from build123d import *

# Parameters (mm, degrees)
ESBO_O1_W                = 300
ESBO_O1_H                = 25
RESSALTO_EXTRUS_O1_DEPTH = 2
ESBO_O2_R                = 2.5
CORTE_EXTRUS_O1_DEPTH    = 3
ESBO_O3_W                = 300
ESBO_O3_H                = 2
RESSALTO_EXTRUS_O2_DEPTH = 25
FILETE1_R                = 3


with BuildPart() as part:
    # Esboço1 → Ressalto-extrusão1 (new body)
    with BuildSketch(Plane(origin=(0, 0, 0), x_dir=(1, 0, 0), z_dir=(0, 1, 0))):
        Rectangle(ESBO_O1_W, ESBO_O1_H)
    extrude(amount=RESSALTO_EXTRUS_O1_DEPTH)

    # Esboço2 → Corte-extrusão1 (cut, through all)
    with BuildSketch(Plane(origin=(0, 2, 0), x_dir=(1, 0, 0), z_dir=(0, 1, 0))):
        with Locations((-130, -2.5)):
            Circle(ESBO_O2_R)
        with Locations((-65, -2.5)):
            Circle(ESBO_O2_R)
        with Locations((0, -2.5)):
            Circle(ESBO_O2_R)
        with Locations((65, -2.5)):
            Circle(ESBO_O2_R)
        with Locations((130, -2.5)):
            Circle(ESBO_O2_R)
    extrude(amount=-CORTE_EXTRUS_O1_DEPTH, mode=Mode.SUBTRACT)

    # Esboço3 → Ressalto-extrusão2 (add)
    with BuildSketch(Plane.XZ):
        with Locations((0, -11.5)):
            Rectangle(ESBO_O3_W, ESBO_O3_H)
    extrude(amount=RESSALTO_EXTRUS_O2_DEPTH)

    # Filete1
    filete1_edges = [part.edges().sort_by_distance(p)[0] for p in [
        (0, 2, -12.5),
    ]]
    fillet(filete1_edges, radius=FILETE1_R)


solid = part.part
Here's how the part is built. I have some questions about the finished solid (model axes, mm). A direction names the side the tool comes from. Coordinates: 2 decimals unless noted, no trailing zeros. Write each loop counter-clockwise with the first axis right and the second up, starting at its lowest first coordinate (ties: lowest second). Pieces come first, ordered by that corner, then holes.
Item 1: If we mould it in two halves opening along X, with no side actions, what happens to faces 1 (the cylindrical face through (-127.615, 1.014, 1.749)), 2 (the flat face through (150, -5, -11)), 3 (the flat face through (-2, 2, -1)), 4 (the flat face through (-150, -5, -11))? For each: +X half, -X half, draft (parallel to the pull), parting line (faces both ways), or undercut.
Item 2: If I drill on line 1 (X direction, y = 0.9, z = 2.5); line 2 (Z direction, x = -92.5, y = -23); line 3 (Y direction, x = 82, z = 0.5), over which ranges is the centre line in solid material (lowest first)?
Item 3: I want a section at D-D on y = -9.25. Write out the boundary of the cut face in (x, z).
Item 4: Will these pins go through, and if not, where does the flat tip stop? pin 1 (6 mm diameter, centred on x = -21, y = -10, fed in from +Z); pin 2 (10 mm diameter, centred on y = -13, z = -4, fed in from +X); pin 3 (6 mm diameter, centred on x = 130, z = 2.5, fed in from -Y).
Item 5: I want a section at A-A on z = 2.5. Write out the boundary of the cut face in (x, y), and give its area (3 significant figures).
Item 6: I want a section at B-B on x = 130. Write out the boundary of the cut face in (y, z).
Item 7: On a 3-axis mill with a long thin cutter (end or side, diameter ignored), from which of +Z, -Z, +X, -X, +Y, -Y can I reach the whole of each face in a straight line? I mean faces 5 (the cylindrical face through (67.385, 1.014, 1.749)), 6 (the flat face through (-2, -12, -10.5)). Say none if no direction works.
Item 8: I want a section at C-C on x = -124.5. Write out the boundary of the cut face in (y, z), and give its area (3 significant figures).
Findings below:
1. face 1: undercut
1. face 2: +X half
1. face 3: draft
1. face 4: -X half
2. line 1: x = -150 to -132.5, -127.5 to -67.5, -62.5 to -2.5, 2.5 to 62.5, 67.5 to 127.5, 132.5 to 150
2. line 2: z = -12.5 to -10.5
2. line 3: y = 0 to 2
3. outline: (-150, -12.5) - (150, -12.5) - (150, -10.5) - (-150, -10.5) - close
4. pin 1: stops at z = -10.5
4. pin 2: passes through
4. pin 3: stops at y = 0
5. outline: (-150, 0) - (-132.5, 0) - (-132.5, 2) - (-150, 2) - close; (-127.5, 0) - (-67.5, 0) - (-67.5, 2) - (-127.5, 2) - close; (-62.5, 0) - (-2.5, 0) - (-2.5, 2) - (-62.5, 2) - close; (2.5, 0) - (62.5, 0) - (62.5, 2) - (2.5, 2) - close; (67.5, 0) - (127.5, 0) - (127.5, 2) - (67.5, 2) - close; (132.5, 0) - (150, 0) - (150, 2) - (132.5, 2) - close
5. area: 550 mm2
6. outline: (-25, -12.5) - (-1, -12.5) arc R3 ccw to (2, -9.5) - (2, 0) - (0, 0) - (0, -10.5) - (-25, -10.5) - close; (0, 5) - (2, 5) - (2, 12.5) - (0, 12.5) - close
7. face 5: +Y, -Y
7. face 6: +Z, +X, -X, -Y
8. outline: (-25, -12.5) - (-1, -12.5) arc R3 ccw to (2, -9.5) - (2, 12.5) - (0, 12.5) - (0, -10.5) - (-25, -10.5) - close
8. area: 98.1 mm2
